from build123d import *

# Parameters (mm, degrees)
F0_R     = 150
F0_W     = 3
F0_H     = 8
F0_W_2   = 13
F0_H_2   = 50
F1_DEPTH = 3
F2_R     = 1.75
F2_W     = 4
F2_H     = 3
F3_DEPTH = 3


with BuildPart() as f1:
    # F0 (on Top) → F1 (new body)
    with BuildSketch(Plane.XY):
        Circle(F0_R)
        with Locations((-142.5, -10)):
            Rectangle(F0_W, F0_H, mode=Mode.SUBTRACT)
        with Locations((142.5, -10)):
            Rectangle(F0_W, F0_H, mode=Mode.SUBTRACT)
        with Locations((-142.5, 10)):
            Rectangle(F0_W, F0_H, mode=Mode.SUBTRACT)
        with Locations((-113.5, 0)):
            Rectangle(F0_W_2, F0_H_2, mode=Mode.SUBTRACT)
        with Locations((113.5, 0)):
            Rectangle(F0_W_2, F0_H_2, mode=Mode.SUBTRACT)
        with Locations((142.5, 10)):
            Rectangle(F0_W, F0_H, mode=Mode.SUBTRACT)
    extrude(amount=-F1_DEPTH)

    # F2 (on face) → F3 (cut, through all)
    with BuildSketch(Plane.XY):
        Polygon((-37.390061, 131.8142), (-41.253764, 130.778924), (-40.477307, 127.881146), (-36.613604, 128.916423), align=None)
        Polygon((-32.21368, 112.495684), (-32.990137, 115.393461), (-36.85384, 114.358185), (-36.077383, 111.460407), align=None)
        with Locations((-32.870019, 122.67258)):
            Circle(F2_R)
        Polygon((-28.886197, 130.986975), (-29.662654, 133.884752), (-33.526358, 132.849476), (-32.7499, 129.951699), align=None)
        Polygon((-25.26273, 117.464013), (-29.126434, 116.428737), (-28.349977, 113.53096), (-24.486273, 114.566236), align=None)
        with Locations((-117.779455, -68)):
            Circle(F2_R)
        Polygon((-108.119201, -64.732051), (-110.717277, -66.232051), (-108.717277, -69.696152), (-106.119201, -68.196152), align=None)
        Polygon((-120.841633, -76.696152), (-122.841633, -73.232051), (-125.439709, -74.732051), (-123.439709, -78.196152), align=None)
        Polygon((-114.717277, -59.303848), (-112.717277, -62.767949), (-110.119201, -61.267949), (-112.119201, -57.803848), align=None)
        Polygon((-127.439709, -71.267949), (-124.841633, -69.767949), (-126.841633, -66.303848), (-129.439709, -67.803848), align=None)
        Polygon((108.717277, -69.696152), (110.717277, -66.232051), (108.119201, -64.732051), (106.119201, -68.196152), align=None)
        Polygon((127.439709, -71.267949), (129.439709, -67.803848), (126.841633, -66.303848), (124.841633, -69.767949), align=None)
        Polygon((112.717277, -62.767949), (114.717277, -59.303848), (112.119201, -57.803848), (110.119201, -61.267949), align=None)
        with Locations((117.779455, -68)):
            Circle(F2_R)
        Polygon((123.439709, -78.196152), (125.439709, -74.732051), (122.841633, -73.232051), (120.841633, -76.696152), align=None)
        with Locations((0, -136)):
            Circle(F2_R)
        with Locations((4, -127.5)):
            Rectangle(F2_W, F2_H)
        with Locations((-4, -127.5)):
            Rectangle(F2_W, F2_H)
        with Locations((4, -144.5)):
            Rectangle(F2_W, F2_H)
        with Locations((-4, -144.5)):
            Rectangle(F2_W, F2_H)
        Polygon((-89.095454, 80.610173), (-86.974134, 78.488853), (-84.145707, 81.31728), (-86.267027, 83.4386), align=None)
        Polygon((-80.610173, 89.095454), (-83.4386, 86.267027), (-81.31728, 84.145707), (-78.488853, 86.974134), align=None)
        with Locations((-89.802561, 89.802561)):
            Circle(F2_R)
        Polygon((-101.11627, 92.630988), (-98.994949, 90.509668), (-96.166522, 93.338095), (-98.287843, 95.459415), align=None)
        Polygon((-95.459415, 98.287843), (-93.338095, 96.166522), (-90.509668, 98.994949), (-92.630988, 101.11627), align=None)
        Polygon((-133.884752, 29.662654), (-130.986975, 28.886197), (-129.951699, 32.7499), (-132.849476, 33.526358), align=None)
        Polygon((-130.778924, 41.253764), (-131.8142, 37.390061), (-128.916423, 36.613604), (-127.881146, 40.477307), align=None)
        Polygon((33.526358, 132.849476), (29.662654, 133.884752), (28.886197, 130.986975), (32.7499, 129.951699), align=None)
        Polygon((40.477307, 127.881146), (41.253764, 130.778924), (37.390061, 131.8142), (36.613604, 128.916423), align=None)
        Polygon((28.349977, 113.53096), (29.126434, 116.428737), (25.26273, 117.464013), (24.486273, 114.566236), align=None)
        Polygon((36.85384, 114.358185), (32.990137, 115.393461), (32.21368, 112.495684), (36.077383, 111.460407), align=None)
        with Locations((32.870019, 122.67258)):
            Circle(F2_R)
        Polygon((93.338095, 96.166522), (95.459415, 98.287843), (92.630988, 101.11627), (90.509668, 98.994949), align=None)
        Polygon((101.11627, 92.630988), (98.287843, 95.459415), (96.166522, 93.338095), (98.994949, 90.509668), align=None)
        Polygon((83.4386, 86.267027), (80.610173, 89.095454), (78.488853, 86.974134), (81.31728, 84.145707), align=None)
        Polygon((89.095454, 80.610173), (86.267027, 83.4386), (84.145707, 81.31728), (86.974134, 78.488853), align=None)
        with Locations((89.802561, 89.802561)):
            Circle(F2_R)
        Polygon((130.778924, 41.253764), (127.881146, 40.477307), (128.916423, 36.613604), (131.8142, 37.390061), align=None)
        Polygon((133.884752, 29.662654), (132.849476, 33.526358), (129.951699, 32.7499), (130.986975, 28.886197), align=None)
    extrude(amount=-F3_DEPTH, mode=Mode.SUBTRACT)


solid = f1.part
Build history of the part. All positions in model axes, mm. Coordinates: 2 decimals unless noted, no trailing zeros. Order: outer loops, then holes, each group sorted by start corner. A loop starts at its lowest first (then second) coordinate and runs counter-clockwise, first axis right, second up. Notation, with made-up numbers: (12, 9) - (43, 9) arc R18 ccw to (43, 20) - close; hole circle Ø5 at (14, -24). An arc over 180 degrees is marked (long way). Write each question's results on one line, items separated by ' | '. Start each with the question number.
Item 1: Band-saw the part on C-C on x = 50.5. Write the cut outline in (y, z), and give its area (3 significant figures).
Item 2: Wall check: probe 1 along Y at (x, z) = (0, -1.85); probe 2 along Y at (x, z) = (112, -0.8); probe 3 along Y at (x, z) = (-79.5, -2.4). Give the ranges that are in metal, low to high. Write a range as [from, to].
Item 3: Band-saw the part on B-B on z = -0.65. State how many separate pieces and enclosed holes the cut face has, and give its area (3 significant figures).
Item 4: Band-saw the part on A-A on y = 0. Write the cut outline in (x, z).
Item 5: Band-saw the part on D-D on y = 106. Write the cut outline in (x, z), and give its area (3 significant figures).
Item 6: Flat gauge pins, fed straight in: pin 1 (1.5 mm diameter, centred on x = 4, z = -2, fed in from +Y); pin 2 (1.5 mm diameter, centred on y = -127, z = -1, fed in from -X); pin 3 (1.5 mm diameter, centred on y = -109, z = -2, fed in from +X); pin 4 (2 mm diameter, centred on x = 0, y = -136, fed in from -Z). Where does each tip first touch, or does it go through?
Numbers:
1) outline: (-141.24, -3) - (141.24, -3) - (141.24, 0) - (-141.24, 0) - close | area: 847 mm^2
2) probe 1: [-150, -137.75], [-134.25, 150] | probe 2: [-99.78, -62.35], [-58.01, -25], [25, 99.78] | probe 3: [-127.2, 85.96], [87.99, 127.2]
3) separate pieces: 1 | enclosed holes: 45 | area: 68,800 mm^2
4) outline: (-150, -3) - (-120, -3) - (-120, 0) - (-150, 0) - close; (-107, -3) - (107, -3) - (107, 0) - (-107, 0) - close; (120, -3) - (150, -3) - (150, 0) - (120, 0) - close
5) outline: (-106.13, -3) - (106.13, -3) - (106.13, 0) - (-106.13, 0) - close | area: 637 mm^2
6) pin 1: y = 149.96 | pin 2: x = -81 | pin 3: x = 103.84 | pin 4: through
